The listing builds one solid part. Answer for the finished solid, in the listing's coordinates (mm). A direction names the side the tool comes from. Round coordinates to 2 decimals unless told otherwise and drop trailing zeros. Order: outer loops, then holes, each group sorted by start corner. A loop starts at its lowest first (then second) coordinate and runs counter-clockwise, first axis right, second up. Notation, with made-up numbers: (84, 52) -> (132, 52) arc R22 ccw to (132, 81) -> close; hole circle Ø5 at (57.5, 5). An arc over 180 degrees is marked (long way). Return JSON: item names as keys, results as strings. Group by question number.
(1) The part is cut by section B-B (y = -5.25). Determine the outline of the cut face in (x, z).
(2) Consider line 1 (X direction, y = -3.5, z = -14.5); line 2 (X direction, y = -5.25, z = -7.75); line 3 (X direction, y = -4.75, z = -18.25). Determine where each line is inside the solid, lowest interval first. Write a range as [from, to].
(3) Determine the mould class of faces 1 (the face through (41.373, -3.131, -12.488)), 2 (the face through (62, -3, -23.952)), 3 (the face through (94.412, -3, -16)) for opening direction X: +X half, -X half, draft (parallel to the pull), parting line (faces both ways), or undercut.
(4) Which of the six approach directions +Z, -Z, +X, -X, +Y, -Y give full straight-line access (tool end or side, diameter ignored) to faces 4 (the face through (15, -3, 0)), 5 (the face through (42, -3, -21.412)), 6 (the face through (42, -6.35, -12)), 7 (the face through (22, -3, -5.08)), 8 (the face through (91.872, -3, -15))?
(5) The part is cut by section A-A (z = -19.5). Determine the outline of the cut face in (x, y).
(6) Each of these flat-tipped pins is pushed along its axis until it touches: pin 1 (1.9 mm diameter, centred on x = 4.5, y = -3.5, fed in from -Z); pin 2 (1 mm diameter, centred on x = 39.5, y = -3, fed in from +Z); pin 3 (8 mm diameter, centred on x = 10.5, z = -5, fed in from -Y); pin 4 (0.8 mm diameter, centred on x = 93, y = -2.5, fed in from +Z). Where does it stop, or does it pass through?
(7) The part is cut by section C-C (z = -12.5). Determine the outline of the cut face in (x, y).
(8) The part is cut by section D-D (x = 55.5). Determine the outline of the cut face in (y, z), plus the area to 3 significant figures.
from build123d import *

# Parameters (mm, degrees)
F0_W     = 14.9098
F0_H     = 2.54
F0_W_2   = 2.54
F0_H_2   = 12.7
F1_DEPTH = 6.35
F2_R     = 0.762


with BuildPart() as f1:
    # F0 (on Front) → F1 (new body)
    with BuildSketch(Plane.XZ):
        Polygon((0, -2.54), (0, 0), (-2.54, 0), (-2.54, -17.78), (0, -17.78), align=None)
        Polygon((29.6418, 0), (0, 0), (0, -2.54), (14.732, -2.54), (29.6418, -2.54), align=None)
        with Locations((22.1869, -3.81)):
            Rectangle(F0_W, F0_H)
        Polygon((32.1818, 0), (29.6418, 0), (29.6418, -2.54), (29.6418, -5.08), (29.6418, -23.9522), (32.1818, -23.9522), (32.1818, -21.4122), (32.1818, -3.81), align=None)
        Polygon((91.8718, -21.4122), (54.6354, -21.4122), (50.8254, -21.4122), (32.1818, -21.4122), (32.1818, -23.9522), (94.4118, -23.9522), (94.4118, -21.4122), align=None)
        with Locations((93.1418, -15.0622)):
            Rectangle(F0_W_2, F0_H_2)
        Polygon((54.6354, -21.4122), (32.1818, 0), (32.1818, -3.81), (50.8254, -21.4122), align=None)
    extrude(amount=F1_DEPTH)

    # F2
    f2_edges = [f1.edges().sort_by_distance(p)[0] for p in [
        (-2.54, -3.175, -17.78),
        (0, -3.175, -17.78),
        (-2.54, -3.175, 0),
        (32.1818, -3.175, -21.4122),
        (14.732, -3.175, -5.08),
        (29.6418, -3.175, -23.9522),
        (94.4118, -3.175, -23.9522),
        (94.4118, -3.175, -8.7122),
        (91.8718, -3.175, -8.7122),
        (91.8718, -3.175, -21.4122),
    ]]
    fillet(f2_edges, radius=F2_R)


solid = f1.part
Answer below:
{
 "1": {"outline": "(-2.54, -17.02) arc R0.76 ccw to (-1.78, -17.78) -> (-0.76, -17.78) arc R0.76 ccw to (0, -17.02) -> (0, -2.54) -> (14.73, -2.54) -> (14.73, -4.32) arc R0.76 ccw to (15.49, -5.08) -> (29.64, -5.08) -> (29.64, -23.19) arc R0.76 ccw to (30.4, -23.95) -> (93.65, -23.95) arc R0.76 ccw to (94.41, -23.19) -> (94.41, -9.47) arc R0.76 ccw to (93.65, -8.71) -> (92.63, -8.71) arc R0.76 ccw to (91.87, -9.47) -> (91.87, -20.65) arc R0.76 cw to (91.11, -21.41) -> (54.64, -21.41) -> (32.18, 0) -> (-1.78, 0) arc R0.76 ccw to (-2.54, -0.76) -> close; hole (32.18, -20.65) arc R0.76 ccw to (32.94, -21.41) -> (50.83, -21.41) -> (32.18, -3.81) -> close"},
 "2": {"line 1": "x = [-2.54, 0], [29.64, 32.18], [43.5, 47.39], [91.87, 94.41]", "line 2": "x = [-2.54, 0], [29.64, 32.18], [36.35, 40.31]", "line 3": "x = [29.64, 32.18], [47.48, 51.32], [91.87, 94.41]"},
 "3": {"face 1": "undercut", "face 2": "draft", "face 3": "+X half"},
 "4": {"face 4": "+Z, +X, -X, +Y, -Y", "face 5": "+Y, -Y", "face 6": "+Z, -Z, +X, -X, -Y", "face 7": "-Z, +Y, -Y", "face 8": "+Z, +Y, -Y"},
 "5": {"outline": "(29.64, -6.35) -> (32.18, -6.35) -> (32.18, 0) -> (29.64, 0) -> close; (48.8, -6.35) -> (52.63, -6.35) -> (52.63, 0) -> (48.8, 0) -> close; (91.87, -6.35) -> (94.41, -6.35) -> (94.41, 0) -> (91.87, 0) -> close"},
 "6": {"pin 1": "stops at z = -2.54", "pin 2": "stops at z = -6.5", "pin 3": "stops at y = -6.35", "pin 4": "stops at z = -8.71"},
 "7": {"outline": "(-2.54, -6.35) -> (0, -6.35) -> (0, 0) -> (-2.54, 0) -> close; (29.64, -6.35) -> (32.18, -6.35) -> (32.18, 0) -> (29.64, 0) -> close; (41.39, -6.35) -> (45.29, -6.35) -> (45.29, 0) -> (41.39, 0) -> close; (91.87, -6.35) -> (94.41, -6.35) -> (94.41, 0) -> (91.87, 0) -> close"},
 "8": {"outline": "(-6.35, -23.95) -> (0, -23.95) -> (0, -21.41) -> (-6.35, -21.41) -> close", "area": "16.1 mm²"}
}
